```python
from build123d import *

# Parameters (mm, degrees)
F0_R     = 2.5
F1_DEPTH = 3.175


with BuildPart() as f1:
    # F0 (on Front) → F1 (new body, symmetric)
    with BuildSketch(Plane.XZ):
        with BuildLine():
            ThreePointArc((12.7, 95.249999), (6.35, 101.600001), (0, 95.249999))
            Line((0, 95.249999), (0, 0))
            Line((0, 0), (3.85, 0))
            ThreePointArc((3.85, 0), (6.35, 2.5), (8.85, 0))
            Line((8.85, 0), (12.7, 0))
            Line((12.7, 0), (12.7, 95.249999))
        make_face()
        with Locations((6.35, 95.250001)):
            Circle(F0_R, mode=Mode.SUBTRACT)
        with BuildLine():
            Line((3.85, 0), (0, 0))
            Line((0, 0), (0, -95.249999))
            ThreePointArc((0, -95.249999), (6.35, -101.599999), (12.7, -95.249999))
            Line((12.7, -95.249999), (12.7, 0))
            Line((12.7, 0), (8.85, 0))
            ThreePointArc((8.85, 0), (6.35, -2.5), (3.85, 0))
        make_face()
        with Locations((6.35, -95.249999)):
            Circle(F0_R, mode=Mode.SUBTRACT)
    extrude(amount=F1_DEPTH, both=True)


solid = f1.part
```
Could you check a few things on this model? Use its own coordinates, in mm. Give positions to 0.01 mm unless a question says otherwise; leave off trailing zeros. Write each loop counter-clockwise with the first axis right and the second up, starting at its lowest first coordinate (ties: lowest second). Pieces come first, ordered by that corner, then holes. Notation, with made-up numbers: (7.25, -8.75) -> (37.25, -8.75) arc R21 cw to (37.25, 2.25) -> close; hole circle Ø11 at (0.5, -15.5). An arc over 180 degrees is marked (long way). Write each question's results on one line, items separated by ' | '.
1. I want a section at A-A, the plane z = 0. Write out the boundary of the cut face in (x, y) (3 decimals).
Check sheet entries:
outline: (0, -3.175) -> (3.85, -3.175) -> (3.85, 3.175) -> (0, 3.175) -> close; (8.85, -3.175) -> (12.7, -3.175) -> (12.7, 3.175) -> (8.85, 3.175) -> close
2. If we mould it in two halves opening along Z, with no side actions, what happens to faces 1 (the cylindrical face through (6.5, 0, 101.6)), 2 (the cylindrical face through (6.02, 0.04, 97.73)), 3 (the flat face through (9, -3.175, 1)), 4 (the cylindrical face through (6.2, 0, -101.6))? For each: released by +Z, released by -Z, zero draft, split by the parting line, or undercut.
Check sheet entries:
face 1: released by +Z | face 2: undercut | face 3: zero draft | face 4: released by -Z
3. Will this pin go through, and if not, where does the flat tip stop? pin 1 Ø4 at (x, z) = (6.35, -95.25) entering from +Y.
Check sheet entries:
pin 1: passes through
4. I want a section at B-B, the plane x = 6.35. Write out the boundary of the cut face in (y, z) (3 decimals), then the cut area to 3 significant figures.
Check sheet entries:
outline: (-3.175, -101.6) -> (3.175, -101.6) -> (3.175, -97.75) -> (-3.175, -97.75) -> close; (-3.175, -92.75) -> (3.175, -92.75) -> (3.175, -2.5) -> (-3.175, -2.5) -> close; (-3.175, 2.5) -> (3.175, 2.5) -> (3.175, 92.75) -> (-3.175, 92.75) -> close; (-3.175, 97.75) -> (3.175, 97.75) -> (3.175, 101.6) -> (-3.175, 101.6) -> close | area: 1,200 mm²
5. I need wall thicknesses on L1, parallel to Z at x = 6.35, y = 0.5; L2, parallel to Z at x = 0.5, y = -1.75; L3, parallel to X at y = 2.25, z = 0. Which ranges of each line are inside material? Lowest first, please.
Check sheet entries:
L1: z = -101.6 to -97.75, -92.75 to -2.5, 2.5 to 92.75, 97.75 to 101.6 | L2: z = -97.72 to 97.72 | L3: x = 0 to 3.85, 8.85 to 12.7
